Model file for the job. Use its own axes, mm. Face numbers are marked on the shaded views. A direction names the side the tool comes from. Coordinates: 2 decimals unless noted, no trailing zeros. Write each loop counter-clockwise with the first axis right and the second up, starting at its lowest first coordinate (ties: lowest second). Pieces come first, ordered by that corner, then holes.
Q1. Pin check, flat tips, straight feed: P1, Ø1.2, axis at y = 52, z = 4, coming from the +X side; P2, Ø3, axis at y = 52, z = -18.5, coming from the -X side; P3, Ø8, axis at x = 16, y = 7, coming from the +Z side. Stop position of each tip, or through.
Q2. Pull direction X, two halves, no side cores. Call the marked faces 1, 2 and 3: released by +X, released by -X, zero draft, split by the parting line, or undercut.
Q3. Drill centre lines: probe 1 along X at (y, z) = (24, -36.5); probe 2 along Z at (x, y) = (31.5, 14). Where is each one in solid material? Low to high.
Q4. Which spindle directions (+Z, -Z, +X, -X, +Y, -Y) get a long thin tool onto all of the face, cutting with end or side? Do the marked faces 4 and 5. Say none if no direction does.
Q5. Band-saw the part on A-A, the plane z = -24.5. Write the cut outline in (x, y).
Q6. Band-saw the part on C-C, the plane y = 21. Write the cut outline in (x, z), plus the area to 4 significant figures.
Q7. Band-saw the part on B-B, the plane x = 0. Write the cut outline in (y, z).
Autodesk Inventor part; units mm, degrees
ref_plane "YZ Plane" through (0, 0, 0) normal (1, 0, 0) x (0, 1, 0)
ref_plane "XZ Plane" through (0, 0, 0) normal (0, 1, 0) x (-1, 0, 0)
ref_plane "XY Plane" through (0, 0, 0) normal (0, 0, 1) x (1, 0, 0)
sketch "Sketch1" plane through (0, 0, 0) normal (0, 1, 0) x (-1, 0, 0)
  line L0 (-37.5, -50) -> (37.5, -50)
  line L1 (37.5, -50) -> (37.5, 50)
  line L2 (37.5, 50) -> (-37.5, 50)
  line L3 (-37.5, 50) -> (-37.5, -50)
  line L4 (-37.5, -50) -> (37.5, 50) construction
  line L5 (37.5, -50) -> (-37.5, 50) construction
  point P0 (0, 0)
  dimension "d0" = 75
  dimension "d1" = 100
extrude "Extrusion1" add sketch "Sketch1" along normal blind 50
sketch "Sketch2" plane through (0, 50, 0) normal (0, 1, 0) x (1, 0, 0)
  line L0 (-37.5, -50) -> (37.5, -50)
  line L1 (-32.5, -50) -> (32.5, -50)
  line L2 (32.5, -50) -> (32.5, 45)
  line L3 (32.5, 45) -> (-32.5, 45)
  line L4 (-32.5, 45) -> (-32.5, -50)
  point P0 (0, 0)
  dimension "d4" = 65
  dimension "d5" = 95
extrude "Extrusion2" cut sketch "Sketch2" against normal blind 50
sketch "Sketch3" plane through (0, 50, 0) normal (0, 1, 0) x (1, 0, 0)
  line L0 (-37.5, -50) -> (-32.5, -50)
  line L1 (-36, -50) -> (-34, -50)
  line L2 (-34, -50) -> (-34, 48.5)
  line L3 (-34, 48.5) -> (-36, 48.5)
  line L4 (-36, 48.5) -> (-36, -50)
  line L5 (-36, 48.5) -> (36, 48.5)
  line L6 (36, 48.5) -> (36, 46.5)
  line L7 (36, 46.5) -> (-36, 46.5)
  line L8 (-36, 46.5) -> (-36, 48.5)
  line L9 (36, 48.5) -> (34, 48.5)
  line L10 (34, 48.5) -> (34, -50)
  line L11 (34, -50) -> (36, -50)
  line L12 (36, -50) -> (36, 48.5)
  point P0 (0, 0)
  dimension "d8" = 2
  dimension "d9" = 98.5
  dimension "d10" = 72
  dimension "d11" = 2
extrude "Extrusion3" add sketch "Sketch3" along normal blind 4
sketch "Sketch4" plane through (36, 50, 50) normal (1, 0, 0) x (0, 0, -1)
  line L0 (0, 0) -> (100, 0)
  line L1 (98.5, 0) -> (98.5, 4)
  line L2 (0, 0) -> (98.5, 0)
  line L3 (98.5, 0) -> (98.5, 4)
  line L4 (98.5, 4) -> (0, 4)
  line L5 (0, 4) -> (0, 0)
  point P0 (50, -50)
extrude "Extrusion4" cut sketch "Sketch4" against normal blind 0.25
sketch "Sketch5" plane through (34, 50, -46.5) normal (-1, 0, 0) x (0, 0, 1)
  line L0 (96.5, 0) -> (96.5, 4)
  line L1 (96.5, 0) -> (0, 0)
  line L2 (96.5, 4) -> (0, 4)
  line L3 (0, 4) -> (0, 0)
  line L4 (0, 0) -> (96.5, 0)
  line L5 (96.5, 0) -> (96.5, 4)
  point P0 (46.5, -50)
extrude "Extrusion5" cut sketch "Sketch5" against normal blind 0.25
sketch "Sketch6" plane through (-36, 50, -48.5) normal (0, 0, -1) x (-1, 0, 0)
  line L0 (-71.75, 4) -> (0, 4)
  line L1 (0, 0) -> (-71.75, 0)
  line L2 (0, 4) -> (-71.75, 4)
  line L3 (-71.75, 4) -> (-71.75, 0)
  line L4 (-71.75, 0) -> (0, 0)
  line L5 (0, 0) -> (0, 4)
  point P0 (-36, -50)
extrude "Extrusion6" cut sketch "Sketch6" against normal blind 0.25
sketch "Sketch7" plane through (-34, 50, 50) normal (1, 0, 0) x (0, 0, -1)
  line L0 (0, 0) -> (0, 4)
  line L1 (0, 4) -> (96.5, 4)
  line L2 (0, 0) -> (96.5, 0)
  line L3 (96.5, 0) -> (96.5, 4)
  line L4 (96.5, 4) -> (0, 4)
  line L5 (0, 4) -> (0, 0)
  point P0 (50, -50)
extrude "Extrusion7" cut sketch "Sketch7" against normal blind 0.25
sketch "Sketch8" plane through (-36, 50, 50) normal (-1, 0, 0) x (0, 0, 1)
  line L0 (0, 4) -> (-96.5, 4)
  line L1 (-98.25, 0) -> (0, 0)
  line L2 (0, 4) -> (-98.25, 4)
  line L3 (-98.25, 4) -> (-98.25, 0)
  line L4 (-98.25, 0) -> (0, 0)
  line L5 (0, 0) -> (0, 4)
  point P0 (-50, -50)
extrude "Extrusion8" cut sketch "Sketch8" against normal blind 0.25
sketch "Sketch9" plane through (-36, 50, -48.25) normal (0, 0, -1) x (-1, 0, 0)
  line L0 (-72, 4) -> (0, 4)
  line L1 (0, 4) -> (0, 0)
  line L2 (0, 0) -> (-72, 0)
  line L3 (-72, 0) -> (-72, 4)
  point P0 (-36, -50)
extrude "Extrusion9" cut sketch "Sketch9" against normal blind 0.25
properties part number "tb3_start_walls_v2"
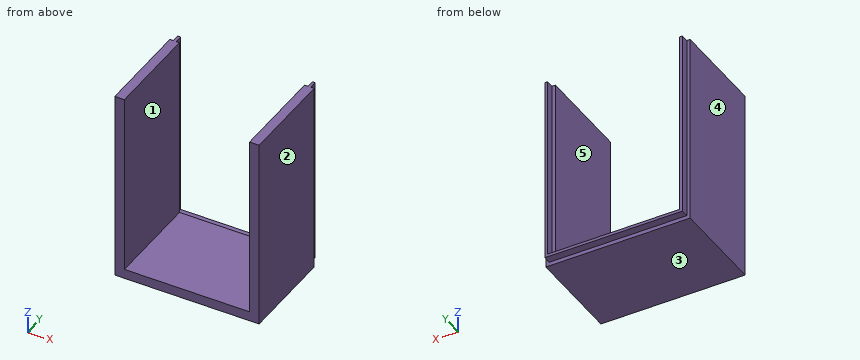
Answer sheet:
1. P1: stops at x = 35.75
1. P2: stops at x = -35.75
1. P3: stops at z = -45
2. face 1: undercut
2. face 2: released by +X
2. face 3: zero draft
3. probe 1: x = -37.5 to -32.5, 32.5 to 37.5
3. probe 2: z = -50 to -45
4. face 4: +Z, -Z, -X, +Y, -Y
4. face 5: +Z, +Y, -Y
5. outline: (-37.5, 0) - (-32.5, 0) - (-32.5, 50) - (-34.25, 50) - (-34.25, 54) - (-35.75, 54) - (-35.75, 50) - (-37.5, 50) - close; (32.5, 0) - (37.5, 0) - (37.5, 50) - (35.75, 50) - (35.75, 54) - (34.25, 54) - (34.25, 50) - (32.5, 50) - close
6. outline: (-37.5, -50) - (37.5, -50) - (37.5, 50) - (32.5, 50) - (32.5, -45) - (-32.5, -45) - (-32.5, 50) - (-37.5, 50) - close
6. area: 1,325 mm2
7. outline: (0, -50) - (50, -50) - (50, -48) - (54, -48) - (54, -46.5) - (50, -46.5) - (50, -45) - (0, -45) - close
